Autodesk Inventor part; units mm, degrees
ref_plane "YZ Plane" through (0, 0, 0) normal (1, 0, 0) x (0, 1, 0)
ref_plane "XZ Plane" through (0, 0, 0) normal (0, 1, 0) x (-1, 0, 0)
ref_plane "XY Plane" through (0, 0, 0) normal (0, 0, 1) x (1, 0, 0)
sketch "Sketch1" plane through (0, 0, 0) normal (1, 0, 0) x (0, 1, 0)
  line L0 (0, 0) -> (709.2052, 0)
  line L1 (774.7, -88.9) -> (0, -88.9)
  line L2 (0, -88.9) -> (0, 0)
  line L3 (774.7, -88.9) -> (909.5108, -88.9) construction
  line L4 (774.7, -88.9) -> (729.4486, 0)
  line L5 (729.4486, 0) -> (709.2052, 0)
extrude "Extrusion1" add sketch "Sketch1" along normal blind 38.1
properties part number "S_2x4x30.5"
Work out the finished part from the listing and answer in its coordinate system (mm). Round coordinates to 2 decimals unless told otherwise and drop trailing zeros. Loops run counter-clockwise (first coordinate to the right, second up) from the corner with the lowest first, then second, coordinate; pieces in that order, holes last. Notation, with made-up numbers: (-19, 79) - (29, 79) arc R29 ccw to (29, 115) - close; hole circle Ø7 at (10, 85.5). An arc over 180 degrees is marked (long way). One line per item, written item: value.
Q1. Find section A-A on x = 20.5. Give the vertices of the cut face in (y, z), and give its area (3 significant figures).
Check values:
outline: (0, -88.9) - (774.7, -88.9) - (729.45, 0) - (0, 0) - close
area: 66,900 mm2
Q2. This flat-tipped pin is pushed along its axis until it touches: pin 1 Ø1.5 at (x, z) = (23, -63.5) entering from +Y. Where does it stop, or does it pass through?
Check values:
pin 1: y = 762.15
Q3. Find section B-B on z = -57. Give the vertices of the cut face in (x, y), and give its area (3 significant figures).
Check values:
outline: (0, 0) - (38.1, 0) - (38.1, 758.46) - (0, 758.46) - close
area: 28,900 mm2
Q4. Straight lines are drawn through the part: probe 1 along Y at (x, z) = (28.5, -13.5); probe 2 along Y at (x, z) = (5, -41.5). For each, find the intervals that lie inside material, in ascending order.
Check values:
probe 1: 0 to 736.32
probe 2: 0 to 750.57
